Source: CAD feature listing. Evaluate the final solid. Frame: model axes, mm. A direction names the side the tool comes from. Round coordinates to 2 decimals unless told otherwise and drop trailing zeros. Loops run counter-clockwise (first coordinate to the right, second up) from the corner with the lowest first, then second, coordinate; pieces in that order, holes last.
(1) First-contact query: pin 1 Ø19 at (x, y) = (55.5, -10.5) entering from +Z; pin 2 Ø12 at (x, y) = (53.5, 23.5) entering from -Z. Flat tips, straight axial feed; report the tip coordinate or a pass-through.
(2) Section A-A, the plane y = -29. Return the cut outline in (x, z), plus the area to 3 significant figures.
(3) Set-up query: faces 1 (the flat face through (38, -1, -1225.096)), 2 (the flat face through (-19.05, -1, 1181)), 3 (the flat face through (-38.1, 1, -1382)). Return all of +Z, -Z, +X, -X, +Y, -Y with unobstructed straight access to the full face (end or side cutting, diameter ignored); none if empty.
(4) Material intervals for probe 1 along Z at (x, y) = (65.5, -36); probe 2 along Z at (x, y) = (-29, 1), sorted ascending.
```python
from build123d import *

# Parameters (mm, degrees)
F1_DEPTH = 76.2
F2_W     = 38.1
F2_H     = 152.4
F3_DEPTH = 317.5


# Not quite as in the source:
# - a feature names something its author has since deleted; it is built from what else it names


with BuildPart() as f1:
    # F0 (on Front) → F1 (new body, symmetric)
    with BuildSketch(Plane.XZ):
        Polygon((-19.05, 1136.65), (-76.2, 1136.1958463669), (-76.2, -1225.0958463669), (76.2, -1225.0958463669), (76.2, 1137.1041536331), (38.1, 1137.1041536331), (19.05, 1136.9527690887), (19.05, 1136.65), align=None)
        Polygon((19.05, 1136.9527690887), (-19.05, 1136.65), (19.05, 1136.65), align=None)
        Polygon((19.05, 1225.0958463669), (-19.05, 1225.0958463669), (-19.05, 1136.65), (19.05, 1136.9527690887), align=None)
    extrude(amount=F1_DEPTH, both=True)

    # F2 (on face) → F3 (join)
    with BuildSketch(Plane(origin=(0, 0, -1225.0958463669), x_dir=(1, 0, 0), z_dir=(0, 0, -1))):
        with Locations((-19.05, 0)):
            Rectangle(F2_W, F2_H)
    extrude(amount=F3_DEPTH)


solid = f1.part
```
Output values:
1. pin 1: stops at z = 1137.1
1. pin 2: stops at z = -1225.1
2. outline: (-76.2, -1225.1) - (-38.1, -1225.1) - (-38.1, -1542.6) - (0, -1542.6) - (0, -1225.1) - (76.2, -1225.1) - (76.2, 1137.1) - (38.1, 1137.1) - (19.05, 1136.95) - (19.05, 1225.1) - (-19.05, 1225.1) - (-19.05, 1136.65) - (-76.2, 1136.2) - close
2. area: 375,000 mm2
3. face 1: -Z, +X, +Y, -Y
3. face 2: +Z, -X, +Y, -Y
3. face 3: -Z, -X, +Y, -Y
4. probe 1: z = -1225.1 to 1137.1
4. probe 2: z = -1542.6 to 1136.57
